The model under review builds one solid part; all positions refer to its coordinate system, in mm. A direction names the side the tool comes from. Coordinates: 2 decimals unless noted, no trailing zeros. Loops run counter-clockwise (first coordinate to the right, second up) from the corner with the lowest first, then second, coordinate; pieces in that order, holes last. Notation, with made-up numbers: (-6.5, -18.5) - (24.5, -18.5) arc R22 ccw to (24.5, 12.5) - close; hole circle Ø9 at (4, -33). An arc over 180 degrees is marked (long way). Answer in a Markdown table with one row per item. Add a question column.
(1) We need section B-B on z = 1.6. Give the number of separate pieces and of enclosed holes in the cut face, plus the area to 3 significant figures.
(2) Mouldability with a two-part tool opening along Y and no side actions: class faces 3 (the flat face through (-11.2, 0.7, 3)), 4 (the cylindrical face through (-43.38, 7.06, 1.48)) as +Y half, -Y half, draft (parallel to the pull), parting line (faces both ways), or undercut.
(3) We need section A-A on x = -15. Write out the cut boundary in (y, z), plus the area to 3 significant figures.
(4) For line 1 along X through (y, z) = (-15, 2.8); line 2 along X through (y, z) = (-4, 0.4); line 3 along Y through (x, z) = (8, 2.7), list the stretches that pass through material, from the lowest coordinate up.
(5) We need section C-C on x = -4.5. Write out the cut boundary in (y, z), plus the area to 3 significant figures.
(6) Machinability: for faces 1 (the flat face through (-11.2, 0.7, 0)), 2 (the flat face through (11.317, -12.009, 1.479)), which of the approach directions +Z, -Z, +X, -X, +Y, -Y give a long, thin tool a straight path to every point of the face, cutting with its end or side? Answer none if there is none.
(7) For P1, Ø1.5, axis at x = 22.5, z = 1.5, coming from the +Y side; P2, Ø1, axis at x = -11, z = 2.5, coming from the +Y side, all flat-tipped, find the tip position at first contact; note any pin that passes through.
from build123d import *

# Parameters (mm, degrees)
F1_R     = 4.58
F1_R_2   = 11
F2_DEPTH = 3


# Not quite as in the source:
# - a feature names something its author has since deleted; it is built from what else it names


with BuildPart() as f2:
    # F1 (on face) → F2 (new body)
    with BuildSketch(Plane.XY):
        Polygon((24.5380218439, 37.3360185584), (9.072936592, 47.5), (-9.0495502624, 43.7515535479), (-27.1720371169, 40.0031070959), (-37.3360185584, 24.5380218439), (-47.5, 9.072936592), (-43.7515535479, -9.0495502624), (-40.0031070959, -27.1720371169), (-24.5380218439, -37.3360185584), (-9.072936592, -47.5), (9.0495502624, -43.7515535479), (27.1720371169, -40.0031070959), (37.3360185584, -24.5380218439), (47.5, -9.072936592), (43.7515535479, 9.0495502624), (40.0031070959, 27.1720371169), align=None)
        with Locations((-6.8599609456, -38.8043858107)):
            Circle(F1_R, mode=Mode.SUBTRACT)
        with Locations((-32.2895692498, -22.5881194432)):
            Circle(F1_R, mode=Mode.SUBTRACT)
        with BuildLine():
            ThreePointArc((-12.4312179995, -20.3423307182), (-22.8394812689, -6.8340101965), (-21.5614159426, 10.1710836469))
            Line((-21.5614159426, 10.1710836469), (-12.4312179995, -20.3423307182))
        make_face(mode=Mode.SUBTRACT)
        with Locations((22.5881194432, -32.2895692498)):
            Circle(F1_R, mode=Mode.SUBTRACT)
        with BuildLine():
            Line((-0.8588934675, -23.8245231224), (23.8395803729, 0.1414483779))
            ThreePointArc((23.8395803729, 0.1414483779), (16.601805328, -17.1092273306), (-0.8588934675, -23.8245231224))
        make_face(mode=Mode.SUBTRACT)
        with Locations((38.8043858107, -6.8599609456)):
            Circle(F1_R, mode=Mode.SUBTRACT)
        with Locations((-38.8043858107, 6.8599609456)):
            Circle(F1_R, mode=Mode.SUBTRACT)
        with Locations((-22.5881194432, 32.2895692498)):
            Circle(F1_R, mode=Mode.SUBTRACT)
        Circle(F1_R_2, mode=Mode.SUBTRACT)
        with BuildLine():
            ThreePointArc((-14.3344307522, 19.0491389572), (5.5013141945, 23.1965760864), (21.3620855471, 10.5833312845))
            Line((21.3620855471, 10.5833312845), (-14.3344307522, 19.0491389572))
        make_face(mode=Mode.SUBTRACT)
        with Locations((32.2895692498, 22.5881194432)):
            Circle(F1_R, mode=Mode.SUBTRACT)
        with Locations((6.8599609456, 38.8043858107)):
            Circle(F1_R, mode=Mode.SUBTRACT)
        with BuildLine():
            Line((-14.3344307522, 19.0491389572), (21.3620855471, 10.5833312845))
            ThreePointArc((21.3620855471, 10.5833312845), (5.5013141945, 23.1965760864), (-14.3344307522, 19.0491389572))
        make_face()
    extrude(amount=F2_DEPTH)


solid = f2.part
Outcome:
| question | item | result |
|---|---|---|
| 1 | separate pieces | 1 |
| 1 | enclosed holes | 11 |
| 1 | area | 5,400 mm² |
| 2 | face 3 | draft |
| 2 | face 4 | undercut |
| 3 | outline | (-43.6, 0) - (-18.53, 0) - (-18.53, 3) - (-43.6, 3) - close; (-11.76, 0) - (42.52, 0) - (42.52, 3) - (-11.76, 3) - close |
| 3 | area | 238 mm² |
| 4 | line 1 | -42.52 to -18.53, -14.03 to 8.24, 18.53 to 43.6 |
| 4 | line 2 | -44.8 to -23.5, -17.32 to -10.25, 10.25 to 19.57, 23.5 to 35.23, 42.38 to 46.45 |
| 4 | line 3 | -43.97 to -22.46, -15.23 to -7.55, 7.55 to 34.37, 43.24 to 47.28 |
| 5 | outline | (-46.55, 0) - (-42.73, 0) - (-42.73, 3) - (-46.55, 3) - close; (-34.88, 0) - (-10.04, 0) - (-10.04, 3) - (-34.88, 3) - close; (10.04, 0) - (44.69, 0) - (44.69, 3) - (10.04, 3) - close |
| 5 | area | 190 mm² |
| 6 | face 1 | -Z, +X, -X, +Y, -Y |
| 6 | face 2 | +Z, -Z |
| 7 | P1 | y = 39.17 |
| 7 | P2 | y = 43.45 |
